Model file for the job. Use its own axes, mm. A direction names the side the tool comes from. Coordinates: 2 decimals unless noted, no trailing zeros. Write each loop counter-clockwise with the first axis right and the second up, starting at its lowest first coordinate (ties: lowest second). Pieces come first, ordered by that corner, then holes. Notation, with made-up numbers: M -4,53 L 37,53 A26 cw 37,76 Z; hole C 73.25,83 d2. An arc over 180 degrees is marked long. Answer in a Markdown table with one row per item. Add a question column.
```python
from build123d import *

# Parameters (mm, degrees)
BOSS_EXTRUDE1_DEPTH = 21
FILLET1_R           = 1


with BuildPart() as part:
    # Sketch1 → Boss-Extrude1 (new body)
    with BuildSketch(Plane(origin=(0, 0, 0), x_dir=(1, 0, 0), z_dir=(0, 1, 0))):
        Polygon((-10.5, 0), (-20.5, 0), (-20.5, 2), (-12.5, 2), (-12.5, 8), (12.5, 8), (12.5, 2), (20.5, 2), (20.5, 0), (10.5, 0), (10.5, 6), (-10.5, 6), align=None)
    extrude(amount=BOSS_EXTRUDE1_DEPTH)

    # Fillet1
    fillet1_edges = [part.edges().sort_by_distance(p)[0] for p in [
        (-12.5, 10.5, -8),
        (12.5, 10.5, -8),
    ]]
    fillet(fillet1_edges, radius=FILLET1_R)


solid = part.part
```
1) Two-plate mould, pull along X, no slides. Class faces 1 (the face through (10.5, 10, -3)), 2 (the face through (-15, 10, 0)), 3 (the face through (-20.5, 10, -1)): released by +X, released by -X, zero draft, split by the parting line, or undercut.
2) Which spindle directions (+Z, -Z, +X, -X, +Y, -Y) get a long thin tool onto all of the face, cutting with end or side? Do faces 4 (the face through (0, 10, -6)), 5 (the face through (-12.5, 10, -4)), 6 (the face through (16, 10, -2)). Say none if no direction does.
3) Drill centre lines: probe 1 along X at (y, z) = (19, -4); probe 2 along X at (y, z) = (3, -0.5); probe 3 along Z at (x, y) = (6, 3.25). Where is each one in solid material? Low to high.
4) Flat gauge pins, fed straight in: pin 1 Ø2.5 at (y, z) = (10, -4) entering from -X; pin 2 Ø6.5 at (x, y) = (-17.5, 6) entering from -Z; pin 3 Ø6.5 at (x, y) = (-0.5, 7) entering from +Z; pin 4 Ø1.5 at (x, z) = (-8, -5) entering from -Y. Where does each tip first touch, or does it go through?
5) Slice it at B-B (y = 10). Give the cut face in (x, z).
6) Slice it at C-C (x = -16). Give the cut face in (y, z).
7) Slice it at A-A (z = -3). Give the cut face in (x, y), then the cut area to 3 significant figures.
Ans:
| question | item | result |
|---|---|---|
| 1 | face 1 | undercut |
| 1 | face 2 | zero draft |
| 1 | face 3 | released by -X |
| 2 | face 4 | +Z, +Y, -Y |
| 2 | face 5 | -Z, -X, +Y, -Y |
| 2 | face 6 | -Z, +X, +Y, -Y |
| 3 | probe 1 | x = -12.5 to -10.5, 10.5 to 12.5 |
| 3 | probe 2 | x = -20.5 to -10.5, 10.5 to 20.5 |
| 3 | probe 3 | z = -8 to -6 |
| 4 | pin 1 | stops at x = -12.5 |
| 4 | pin 2 | stops at z = -2 |
| 4 | pin 3 | stops at z = -6 |
| 4 | pin 4 | passes through |
| 5 | outline | M -20.5,-2 L -12.5,-2 L -12.5,-7 A1 ccw -11.5,-8 L 11.5,-8 A1 ccw 12.5,-7 L 12.5,-2 L 20.5,-2 L 20.5,0 L 10.5,0 L 10.5,-6 L -10.5,-6 L -10.5,0 L -20.5,0 Z |
| 6 | outline | M 0,-2 L 21,-2 L 21,0 L 0,0 Z |
| 7 | outline | M -12.5,0 L -10.5,0 L -10.5,21 L -12.5,21 Z; M 10.5,0 L 12.5,0 L 12.5,21 L 10.5,21 Z |
| 7 | area | 84.0 mm2 |
